The listing builds one solid part. Answer for the finished solid, in the listing's coordinates (mm). Round coordinates to 2 decimals unless told otherwise and drop trailing zeros. Order: outer loops, then holes, each group sorted by start corner. A loop starts at its lowest first (then second) coordinate and runs counter-clockwise, first axis right, second up. Notation, with made-up numbers: (-8, 8.25) -> (12, 8.25) arc R29 ccw to (12, 40.25) -> close; hole circle Ø9 at (-17.5, 31.25). An arc over 180 degrees is marked (long way). Answer in a Markdown table with one row per item. Add a question column.
```python
from build123d import *

# Parameters (mm, degrees)
SKETCH1_W           = 160
SKETCH1_H           = 160
SKETCH1_R           = 2.2
SKETCH1_R_2         = 4.25
SKETCH1_R_3         = 2.75
SKETCH1_R_4         = 2.25
BOSS_EXTRUDE1_DEPTH = 5


with BuildPart() as part:
    # Sketch1 → Boss-Extrude1 (new body)
    with BuildSketch(Plane(origin=(0, 0, 0), x_dir=(1, 0, 0), z_dir=(0, 1, 0))):
        Rectangle(SKETCH1_W, SKETCH1_H)
        with Locations((48.790367902, 48.790367902)):
            Circle(SKETCH1_R, mode=Mode.SUBTRACT)
        with Locations((48.790367902, -48.790367902)):
            Circle(SKETCH1_R, mode=Mode.SUBTRACT)
        with Locations((-48.790367902, -48.790367902)):
            Circle(SKETCH1_R, mode=Mode.SUBTRACT)
        with Locations((-48.790367902, 48.790367902)):
            Circle(SKETCH1_R, mode=Mode.SUBTRACT)
        Circle(SKETCH1_R_2, mode=Mode.SUBTRACT)
        with Locations((18.272421355, -0.571625498)):
            Circle(SKETCH1_R_3, mode=Mode.SUBTRACT)
        with Locations((-18.227578645, -0.571625498)):
            Circle(SKETCH1_R_3, mode=Mode.SUBTRACT)
        with Locations((0, 65)):
            Circle(SKETCH1_R, mode=Mode.SUBTRACT)
        with Locations((65, 0)):
            Circle(SKETCH1_R, mode=Mode.SUBTRACT)
        with Locations((0, -65)):
            Circle(SKETCH1_R, mode=Mode.SUBTRACT)
        with Locations((-65, 0)):
            Circle(SKETCH1_R, mode=Mode.SUBTRACT)
        with Locations((-65, 65)):
            Circle(SKETCH1_R_4, mode=Mode.SUBTRACT)
        with Locations((65, 65)):
            Circle(SKETCH1_R_4, mode=Mode.SUBTRACT)
        with Locations((65, -65)):
            Circle(SKETCH1_R_4, mode=Mode.SUBTRACT)
        with Locations((-65, -65)):
            Circle(SKETCH1_R_4, mode=Mode.SUBTRACT)
    extrude(amount=BOSS_EXTRUDE1_DEPTH)


solid = part.part
```
Item 1: The part is cut by section B-B, the plane z = -65. Give the vertices of the cut face in (x, y).
Item 2: Find the intervals of material crossed by probe 1 along X at (y, z) = (3.55, -65); probe 2 along Z at (x, y) = (0, 3.2), in increasing order. Write a range as [from, to].
Item 3: The part is cut by section A-A, the plane x = 65. Give the vertices of the cut face in (y, z).
Item 4: For a pull along X with two mould halves and no side action, classify faces 1 (the face through (-1, 2, -80)), 2 (the face through (63.214, 2.465, -63.631)), 3 (the face through (-50.99, 2.46, -48.89)), 4 (the face through (-80, 2, 1)) as released by +X, released by -X, zero draft, split by the parting line, or undercut.
Resolved:
| question | item | result |
|---|---|---|
| 1 | outline | (-80, 0) -> (-67.25, 0) -> (-67.25, 5) -> (-80, 5) -> close; (-62.75, 0) -> (-2.2, 0) -> (-2.2, 5) -> (-62.75, 5) -> close; (2.2, 0) -> (62.75, 0) -> (62.75, 5) -> (2.2, 5) -> close; (67.25, 0) -> (80, 0) -> (80, 5) -> (67.25, 5) -> close |
| 2 | probe 1 | [-80, -67.25], [-62.75, -2.2], [2.2, 62.75], [67.25, 80] |
| 2 | probe 2 | [-80, -67.2], [-62.8, -4.25], [4.25, 62.8], [67.2, 80] |
| 3 | outline | (0, -80) -> (5, -80) -> (5, -67.25) -> (0, -67.25) -> close; (0, -62.75) -> (5, -62.75) -> (5, -2.2) -> (0, -2.2) -> close; (0, 2.2) -> (5, 2.2) -> (5, 62.75) -> (0, 62.75) -> close; (0, 67.25) -> (5, 67.25) -> (5, 80) -> (0, 80) -> close |
| 4 | face 1 | zero draft |
| 4 | face 2 | undercut |
| 4 | face 3 | undercut |
| 4 | face 4 | released by -X |
